from build123d import *

# Parameters (mm, degrees)
F0_W            = 210
F0_H            = 240
F1_DEPTH        = 10
F3_DEPTH        = 1.5
F4_W            = 180
F4_H            = 180
F5_DEPTH        = 3
F7_DEPTH        = 3
F9_DEPTH        = 3
F11_DEPTH       = 3
F13_DEPTH       = 2
F15_D           = 5.5
F17_D           = 4.4
F17_CBORE_D     = 8.25
F17_CBORE_DEPTH = 4
F18_D           = 2.5
F18_DEPTH       = 8
F18_TIP         = 0.7510757738
F20_D           = 4.4
F20_DEPTH       = 5
F20_TIP         = 1.3218933619
F22_D           = 4.2
F22_DEPTH       = 5
F22_CBORE_D     = 10
F22_CBORE_DEPTH = 0.7
F22_TIP         = 1.2618073
F23_SIZE        = 5
F24_R           = 1.5
F25_R           = 2


with BuildPart() as f1:
    # F0 (on Top) → F1 (new body)
    with BuildSketch(Plane.XY):
        Rectangle(F0_W, F0_H)
    extrude(amount=F1_DEPTH)

    # F2 (on face) → F3 (cut)
    with BuildSketch(Plane.XY.offset(10)):
        with BuildLine():
            Line((102.5, -94.5), (102.5, 94.5))
            ThreePointArc((102.5, 94.5), (95.7634559673, 110.7634559673), (79.5, 117.5))
            Line((79.5, 117.5), (-79.5, 117.5))
            ThreePointArc((-79.5, 117.5), (-95.7634559673, 110.7634559673), (-102.5, 94.5))
            Line((-102.5, 94.5), (-102.5, -94.5))
            ThreePointArc((-102.5, -94.5), (-95.7634559673, -110.7634559673), (-79.5, -117.5))
            Line((-79.5, -117.5), (79.5, -117.5))
            ThreePointArc((79.5, -117.5), (95.7634559673, -110.7634559673), (102.5, -94.5))
        make_face()
        with BuildLine():
            ThreePointArc((99.5, -94.5), (93.6421356237, -108.6421356237), (79.5, -114.5))
            Line((79.5, -114.5), (-79.5, -114.5))
            ThreePointArc((-79.5, -114.5), (-93.6421356237, -108.6421356237), (-99.5, -94.5))
            Line((-99.5, -94.5), (-99.5, 94.5))
            ThreePointArc((-99.5, 94.5), (-93.6421356237, 108.6421356237), (-79.5, 114.5))
            Line((-79.5, 114.5), (79.5, 114.5))
            ThreePointArc((79.5, 114.5), (93.6421356237, 108.6421356237), (99.5, 94.5))
            Line((99.5, 94.5), (99.5, -94.5))
        make_face(mode=Mode.SUBTRACT)
    extrude(amount=-F3_DEPTH, mode=Mode.SUBTRACT)

    # F4 (on face) → F5 (cut)
    with BuildSketch(Plane.XY.offset(10)):
        with BuildLine():
            ThreePointArc((95, 92), (94.1213203436, 94.1213203436), (92, 95))
            Line((92, 95), (-92, 95))
            ThreePointArc((-92, 95), (-94.1213203436, 94.1213203436), (-95, 92))
            Line((-95, 92), (-95, -92))
            ThreePointArc((-95, -92), (-94.1213203436, -94.1213203436), (-92, -95))
            Line((-92, -95), (92, -95))
            ThreePointArc((92, -95), (94.1213203436, -94.1213203436), (95, -92))
            Line((95, -92), (95, 92))
        make_face()
        Rectangle(F4_W, F4_H, mode=Mode.SUBTRACT)
    extrude(amount=-F5_DEPTH, mode=Mode.SUBTRACT)

    # F6 (on face) → F7 (cut, through all)
    with BuildSketch(Plane.XY.offset(10)):
        with BuildLine():
            ThreePointArc((68, 36.7157287525), (67.7716385975, 37.8637790496), (67.1213203436, 38.8370490961))
            Line((67.1213203436, 38.8370490961), (38.8370490961, 67.1213203436))
            ThreePointArc((38.8370490961, 67.1213203436), (37.8637790496, 67.7716385975), (36.7157287525, 68))
            Line((36.7157287525, 68), (0, 68))
            Line((0, 68), (-36.7157287525, 68))
            ThreePointArc((-36.7157287525, 68), (-37.8637790496, 67.7716385975), (-38.8370490961, 67.1213203436))
            Line((-38.8370490961, 67.1213203436), (-67.1213203436, 38.8370490961))
            ThreePointArc((-67.1213203436, 38.8370490961), (-67.7716385975, 37.8637790496), (-68, 36.7157287525))
            Line((-68, 36.7157287525), (-68, 0))
            Line((-68, 0), (-68, -36.7157287525))
            ThreePointArc((-68, -36.7157287525), (-67.7716385975, -37.8637790496), (-67.1213203436, -38.8370490961))
            Line((-67.1213203436, -38.8370490961), (-38.8370490961, -67.1213203436))
            ThreePointArc((-38.8370490961, -67.1213203436), (-37.8637790496, -67.7716385975), (-36.7157287525, -68))
            Line((-36.7157287525, -68), (0, -68))
            Line((0, -68), (36.7157287525, -68))
            ThreePointArc((36.7157287525, -68), (37.8637790496, -67.7716385975), (38.8370490961, -67.1213203436))
            Line((38.8370490961, -67.1213203436), (67.1213203436, -38.8370490961))
            ThreePointArc((67.1213203436, -38.8370490961), (67.7716385975, -37.8637790496), (68, -36.7157287525))
            Line((68, -36.7157287525), (68, 0))
            Line((68, 0), (68, 36.7157287525))
        make_face()
        Polygon((-65, -36.7157287525), (-65, 0), (-65, 36.7157287525), (-36.7157287525, 65), (0, 65), (36.7157287525, 65), (65, 36.7157287525), (65, 0), (65, -36.7157287525), (36.7157287525, -65), (0, -65), (-36.7157287525, -65), align=None, mode=Mode.SUBTRACT)
    extrude(amount=-F7_DEPTH, mode=Mode.SUBTRACT)

    # F8 (on face) → F9 (cut, through all)
    with BuildSketch(Plane.XY.offset(10)):
        Polygon((-54, 45.1715728753), (-54, 0), (-54, -45.1715728753), (-40.6715728753, -58.5), (-5.5, -58.5), (-5.5, -54.3), (0, -54.3), (5.5, -54.3), (5.5, -58.5), (40.6715728753, -58.5), (54, -45.1715728753), (54, 0), (54, 45.1715728753), (40.6715728753, 58.5), (5.5, 58.5), (5.5, 54.3), (0, 54.3), (-5.5, 54.3), (-5.5, 58.5), (-40.6715728753, 58.5), align=None)
        Polygon((-51.5, -44.1360389693), (-51.5, 0), (-51.5, 44.1360389693), (-45.1360389693, 50.5), (0, 50.5), (45.1360389693, 50.5), (51.5, 44.1360389693), (51.5, 0), (51.5, -44.1360389693), (45.1360389693, -50.5), (0, -50.5), (-45.1360389693, -50.5), align=None, mode=Mode.SUBTRACT)
    extrude(amount=-F9_DEPTH, mode=Mode.SUBTRACT)

    # F10 (on face) → F11 (cut, through all)
    with BuildSketch(Plane.XY.offset(10)):
        with BuildLine():
            ThreePointArc((-45.7, 42.75), (-46.95, 44), (-48.2, 42.75))
            Line((-48.2, 42.75), (-48.2, -42.75))
            ThreePointArc((-48.2, -42.75), (-46.95, -44), (-45.7, -42.75))
            Line((-45.7, -42.75), (-45.7, 42.75))
        make_face()
        with BuildLine():
            ThreePointArc((45.7, -42.75), (46.95, -44), (48.2, -42.75))
            Line((48.2, -42.75), (48.2, 42.75))
            ThreePointArc((48.2, 42.75), (46.95, 44), (45.7, 42.75))
            Line((45.7, 42.75), (45.7, -42.75))
        make_face()
    extrude(amount=-F11_DEPTH, mode=Mode.SUBTRACT)

    # F12 (on face) → F13 (cut)
    with BuildSketch(Plane.XY.offset(10)):
        with BuildLine():
            Line((-36.5, -47.5), (36.5, -47.5))
            ThreePointArc((36.5, -47.5), (40.7426406871, -45.7426406871), (42.5, -41.5))
            Line((42.5, -41.5), (42.5, 41.5))
            ThreePointArc((42.5, 41.5), (40.7426406871, 45.7426406871), (36.5, 47.5))
            Line((36.5, 47.5), (-36.5, 47.5))
            ThreePointArc((-36.5, 47.5), (-40.7426406871, 45.7426406871), (-42.5, 41.5))
            Line((-42.5, 41.5), (-42.5, -41.5))
            ThreePointArc((-42.5, -41.5), (-40.7426406871, -45.7426406871), (-36.5, -47.5))
        make_face()
    extrude(amount=-F13_DEPTH, mode=Mode.SUBTRACT)

    # F15 (through all)
    with Locations(Plane.XY.offset(8)):
        with Locations((-9.5, 0), (9.5, 0)):
            Hole(F15_D / 2)

    # F17 (through all)
    with Locations(Plane.XY.offset(10)):
        with Locations((0, 59.65), (59.5, 0), (0, -59.65), (-59.5, 0)):
            CounterBoreHole(F17_D / 2, F17_CBORE_D / 2, F17_CBORE_DEPTH)

    # F18
    with Locations(Plane.XY.offset(10)):
        with Locations((-80, 100), (-67.5, 103), (80, 100), (-80, -100), (80, -100), (67.5, -103)):
            Hole(F18_D / 2, depth=F18_DEPTH)
            with Locations((0, 0, -(F18_DEPTH + F18_TIP / 2))):  # 118° drill point
                Cone(0, F18_D / 2, F18_TIP, mode=Mode.SUBTRACT)

    # F20
    with Locations(Plane.XY.offset(7)):
        with Locations((-92.5, 0)):
            Hole(F20_D / 2, depth=F20_DEPTH)
            with Locations((0, 0, -(F20_DEPTH + F20_TIP / 2))):  # 118° drill point
                Cone(0, F20_D / 2, F20_TIP, mode=Mode.SUBTRACT)

    # F22
    with Locations(Plane(origin=(0, 0, 0), x_dir=(1, 0, 0), z_dir=(0, 0, -1))):
        with Locations((-17.5, -57.5), (17.5, 57.5)):
            CounterBoreHole(F22_D / 2, F22_CBORE_D / 2, F22_CBORE_DEPTH, depth=F22_DEPTH)
            with Locations((0, 0, -(F22_DEPTH + F22_TIP / 2))):  # 118° drill point
                Cone(0, F22_D / 2, F22_TIP, mode=Mode.SUBTRACT)

    # F23
    f23_edges = [f1.edges().sort_by_distance(p)[0] for p in [
        (-105, 120, 5),
        (105, 120, 5),
        (-105, -120, 5),
        (105, -120, 5),
    ]]
    chamfer(f23_edges, length=F23_SIZE)

    # F24
    f24_edges = [f1.edges().sort_by_distance(p)[0] for p in [
        (-5.5, 58.5, 8.5),
        (5.5, 58.5, 8.5),
        (5.5, -58.5, 8.5),
        (-5.5, -58.5, 8.5),
    ]]
    fillet(f24_edges, radius=F24_R)

    # F25
    f25_edges = [f1.edges().sort_by_distance(p)[0] for p in [
        (40.671573, 58.5, 8.5),
        (-40.671573, 58.5, 8.5),
        (-54, 45.171573, 8.5),
        (-54, -45.171573, 8.5),
        (-40.671573, -58.5, 8.5),
        (40.671573, -58.5, 8.5),
        (54, -45.171573, 8.5),
        (54, 45.171573, 8.5),
    ]]
    fillet(f25_edges, radius=F25_R)


solid = f1.part
The model under review builds one solid part; all positions refer to its coordinate system, in mm. A direction names the side the tool comes from. Round coordinates to 2 decimals unless told otherwise and drop trailing zeros. Order: outer loops, then holes, each group sorted by start corner. A loop starts at its lowest first (then second) coordinate and runs counter-clockwise, first axis right, second up. Notation, with made-up numbers: (47, 1) -> (54, 1) arc R6 cw to (54, 9) -> close; hole circle Ø7 at (-28.5, -38.5). An arc over 180 degrees is marked (long way). Use CSV: the item, a comma, the result in double quotes. Start each with the question number.
(1) Mouldability with a two-part tool opening along X and no side actions: class faces 3 (the face through (5, -57, 10)), 4 (the face through (52.78, -53.18, 8.52)), 5 (the face through (-105, -2, 5)), 6 (the face through (47.25, -51.92, 8.52)) as pulls with the +X half, pulls with the -X half, needs draft (parallel to the pull), parting line crosses it, or undercut.
(2) Consider section A-A on x = -76. Write out the cut boundary in (y, z), and give its area (3 significant figures).
(3) Tool access review of faces 1 (the face through (93.797, -108.486, 9.26)), 2 (the face through (-12.04, -1.05, 3.94)): name each direction out of +Z, -Z, +X, -X, +Y, -Y from which nothing blocks a thin tool from reaching the whole face with its end or side.
(4) Wall thickness on probe 1 along Y at (x, z) = (-71.5, 8.25); probe 2 along Y at (x, z) = (9.5, 4.75); probe 3 along Y at (x, z) = (17.5, 0.45): over which ranges is each line inside the solid? List them lowest first. Write a range as from..to.
(5) Insertion check: pin 1 (3.5 mm diameter, centred on x = 0, y = 59.65, fed in from +Z); pin 2 (3 mm diameter, centred on x = 18.5, y = -57, fed in from -Z). Each pin has a flat end and moves straight along its axis. Give the tip position at first contact, or say it passes through.
Responses:
1,face 3,"needs draft"
1,face 4,"undercut"
1,face 5,"pulls with the -X half"
1,face 6,"undercut"
2,outline,"(-120, 0) -> (120, 0) -> (120, 10) -> (117.5, 10) -> (117.5, 8.5) -> (114.5, 8.5) -> (114.5, 10) -> (95, 10) -> (95, 7) -> (90, 7) -> (90, 10) -> (-90, 10) -> (-90, 7) -> (-95, 7) -> (-95, 10) -> (-114.5, 10) -> (-114.5, 8.5) -> (-117.5, 8.5) -> (-117.5, 10) -> (-120, 10) -> close"
2,area,"2,360 mm²"
3,face 1,"+Z"
3,face 2,"+Z, -Z"
4,probe 1,"-120..-95, -90..90, 95..120"
4,probe 2,"-120..-2.75, 2.75..120"
4,probe 3,"-120..-62.5, -52.5..120"
5,pin 1,"through"
5,pin 2,"z = 0.7"
